Here's the drawing with two shaded views (mm, measured from the low corner). I have some questions. Round coordinates to 2 decimals unless told otherwise and drop trailing zeros. Order: outer loops, then holes, each group sorted by start corner. A loop starts at its lowest first (then second) coordinate and runs counter-clockwise, first axis right, second up. Notation, with made-up numbers: (52, -6) -> (109, -6) arc R18 cw to (109, 4) -> close; hole circle Ø11 at (85, -30.5). An arc over 180 degrees is marked (long way). Answer in a Markdown table with one row per item.
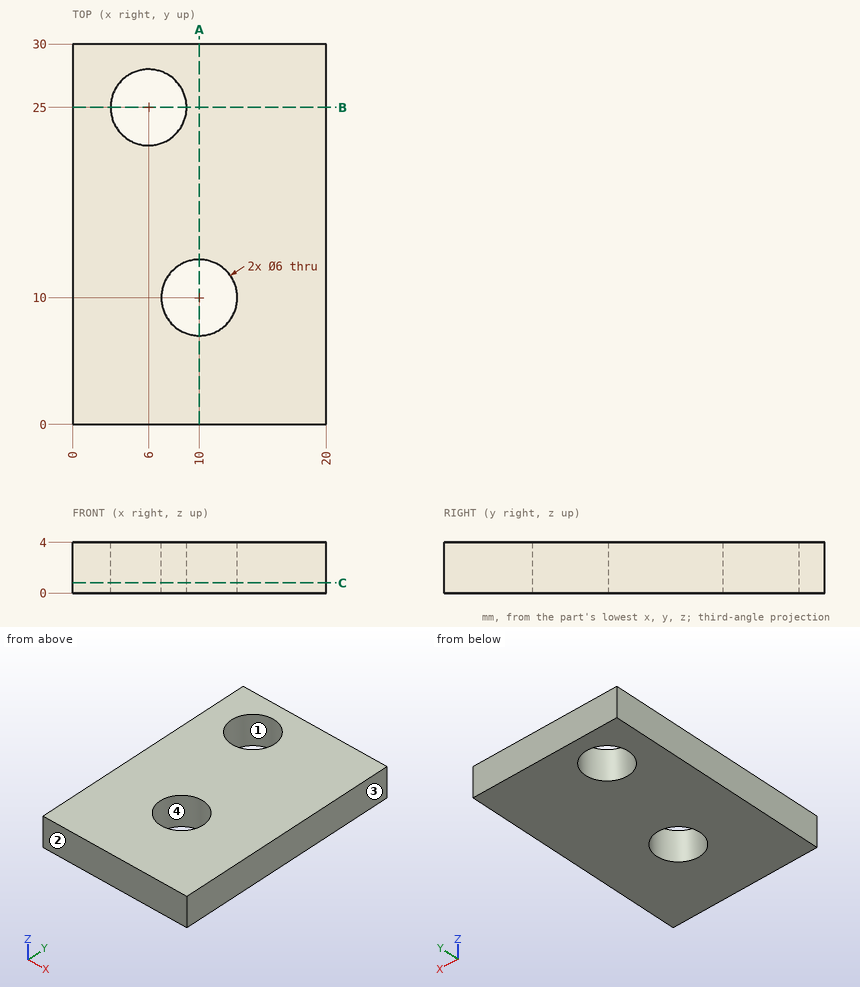
1. Please list where these lines run through material, in increasing order: line 1 along Y through (x, z) = (10, 1.85); line 2 along Y through (x, z) = (6, 2.8); line 3 along X through (y, z) = (25, 1.6).
Numbers:
| item | result |
|---|---|
| line 1 | y = 0 to 7, 13 to 30 |
| line 2 | y = 0 to 22, 28 to 30 |
| line 3 | x = 0 to 3, 9 to 20 |
2. For pin 1 Ø5.5 at (x, y) = (6, 25) entering from -Z, with a flat end and sliding along its axis, tell me the tip position at first contact or that it passes through.
Numbers:
| item | result |
|---|---|
| pin 1 | passes through |
3. We'd pull the mould along X, two halves only. Please class the marked faces 1, 2, 3 and 4: released by +X, released by -X, zero draft, split by the parting line, or undercut.
Numbers:
| item | result |
|---|---|
| face 1 | undercut |
| face 2 | zero draft |
| face 3 | released by +X |
| face 4 | undercut |
4. Suppose I cut it at B-B on y = 25. Write out the boundary of the cut face in (x, z), then the cut area to 3 significant figures.
Numbers:
| item | result |
|---|---|
| outline | (0, 0) -> (3, 0) -> (3, 4) -> (0, 4) -> close; (9, 0) -> (20, 0) -> (20, 4) -> (9, 4) -> close |
| area | 56.0 mm2 |
5. Suppose I cut it at A-A on x = 10. Write out the boundary of the cut face in (y, z).
Numbers:
| item | result |
|---|---|
| outline | (0, 0) -> (7, 0) -> (7, 4) -> (0, 4) -> close; (13, 0) -> (30, 0) -> (30, 4) -> (13, 4) -> close |
6. Suppose I cut it at C-C on z = 0.8. Write out the boundary of the cut face in (x, y).
Numbers:
| item | result |
|---|---|
| outline | (0, 0) -> (20, 0) -> (20, 30) -> (0, 30) -> close; hole circle Ø6 at (6, 25); hole circle Ø6 at (10, 10) |
